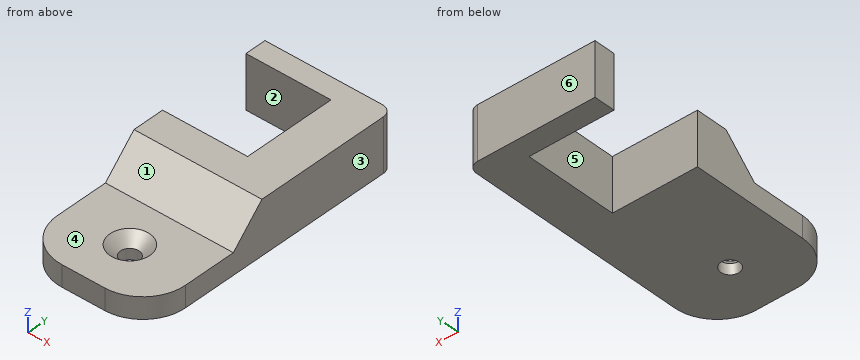
```python
from build123d import *

# Parameters (mm, degrees)
PAD_DEPTH    = 10
SKETCH001_W  = 24.062258
SKETCH001_H  = 24.062258
PAD001_DEPTH = 4
SKETCH002_R  = 1.75
POCKET_DEPTH = 4.001
CHAMFER_SIZE = 2
FILLET_R     = 8
FILLET001_R  = 2
PAD002_DEPTH = 24.062258


with BuildPart() as part:
    # Sketch → Pad (new body)
    with BuildSketch(Plane.XY):
        Polygon((0, 8.75), (0, 12.75), (24.062258, 12.75), (24.062258, -14.75), (0, -14.75), (0, -8.75), (16, -8.75), (16, 8.75), align=None)
    extrude(amount=PAD_DEPTH)

    # Sketch001 (on Face9 of Pad) → Pad001 (join)
    with BuildSketch(Plane(origin=(0, 0, 0), x_dir=(1, 0, 0), z_dir=(0, 0, -1))):
        with Locations((12.031129, 26.781129)):
            Rectangle(SKETCH001_W, SKETCH001_H)
    extrude(amount=-PAD001_DEPTH)

    # Sketch002 (on Face15 of Pad001) → Pocket (cut, through all)
    with BuildSketch(Plane.XY.offset(4)):
        with Locations((12.031129, -29.039748)):
            Circle(SKETCH002_R)
    extrude(amount=-POCKET_DEPTH, mode=Mode.SUBTRACT)

    # Chamfer
    chamfer_edges = [part.edges().sort_by_distance(p)[0] for p in [
        (10.281129, -29.039748, 4),
    ]]
    chamfer(chamfer_edges, length=CHAMFER_SIZE)

    # Fillet
    fillet_edges = [part.edges().sort_by_distance(p)[0] for p in [
        (0, -38.812258, 2),
        (24.062258, -38.812258, 2),
    ]]
    fillet(fillet_edges, radius=FILLET_R)

    # Fillet001
    fillet001_edges = [part.edges().sort_by_distance(p)[0] for p in [
        (24.062258, 12.75, 5),
    ]]
    fillet(fillet001_edges, radius=FILLET001_R)

    # Sketch003 (on Face12 of Fillet001) → Pad002 (join)
    with BuildSketch(Plane.YZ.offset(24.062258)):
        Polygon((-20.75, 4), (-14.75, 10), (-14.75, 4), align=None)
    extrude(amount=-PAD002_DEPTH)


solid = part.part
```
Geometry check sheet. Reference: the model listing, model coordinates, mm. Face numbers are marked on the shaded views. A direction names the side the tool comes from. Give positions to 0.01 mm unless a question says otherwise; leave off trailing zeros. Write each loop counter-clockwise with the first axis right and the second up, starting at its lowest first coordinate (ties: lowest second). Pieces come first, ordered by that corner, then holes. Notation, with made-up numbers: (-1.75, 65) - (50.25, 65) arc R9 ccw to (50.25, 72) - close; hole circle Ø1 at (81.5, 76). An arc over 180 degrees is marked (long way). Use a Markdown table: item, result.
Q1. Set-up check for the marked faces 4, 5 and 6: record each of +Z, -Z, +X, -X, +Y, -Y from which the full face is reachable in a straight line by a thin tool's end or side.
Computed:
| item | result |
|---|---|
| face 4 | +Z, +X, -X, -Y |
| face 5 | +Z, -Z, -X |
| face 6 | +Z, -Z, +X, -X, +Y |
Q2. Section check B-B, the plane x = 3.5. Enter the section's corners in (y, z).
Computed:
| item | result |
|---|---|
| outline | (-37.43, 0) - (-8.75, 0) - (-8.75, 10) - (-14.75, 10) - (-20.75, 4) - (-37.43, 4) - close; (8.75, 0) - (12.75, 0) - (12.75, 10) - (8.75, 10) - close |
Q3. Section check D-D, the plane y = -16. Enter the section's corners in (x, z), then the cut area to 3 significant figures.
Computed:
| item | result |
|---|---|
| outline | (0, 0) - (24.06, 0) - (24.06, 8.75) - (0, 8.75) - close |
| area | 211 mm² |
Q4. Draft check along Y on the marked faces 1, 2 and 3. Enter one of: pulls with the +Y half, pulls with the -Y half, needs draft (parallel to the pull), parting line crosses it, or undercut.
Computed:
| item | result |
|---|---|
| face 1 | pulls with the -Y half |
| face 2 | undercut |
| face 3 | needs draft |
Q5. Section check C-C, the plane z = 1.5. Enter the section's corners in (x, y), then the cut area to 3 significant figures.
Computed:
| item | result |
|---|---|
| outline | (0, -30.81) arc R8 ccw to (8, -38.81) - (16.06, -38.81) arc R8 ccw to (24.06, -30.81) - (24.06, 10.75) arc R2 ccw to (22.06, 12.75) - (0, 12.75) - (0, 8.75) - (16, 8.75) - (16, -8.75) - (0, -8.75) - close; hole circle Ø3.5 at (12.03, -29.04) |
| area | 923 mm² |
Q6. Section check A-A, the plane z = 8. Enter the section's corners in (x, y), then the cut area to 3 significant figures.
Computed:
| item | result |
|---|---|
| outline | (0, -16.75) - (24.06, -16.75) - (24.06, 10.75) arc R2 ccw to (22.06, 12.75) - (0, 12.75) - (0, 8.75) - (16, 8.75) - (16, -8.75) - (0, -8.75) - close |
| area | 429 mm² |
Q7. Go/stop test with flat-tipped pins: P1, Ø4.5, axis at x = 12.03, y = -29.04, coming from the +Z side; P2, Ø5, axis at x = 12, z = 7, coming from the -Y side; P3, Ø1.5, axis at x = 18, y = -19.5, coming from the +Z side. Record where each tip stops, or that it passes through.
Computed:
| item | result |
|---|---|
| P1 | stops at z = 2.5 |
| P2 | stops at y = -20.25 |
| P3 | stops at z = 6 |
Q8. Thickness scan on L1, parallel to Y at x = 14, z = 3; L2, parallel to X at y = 5.5, z = 1.5; L3, parallel to Z at x = 6.25, y = -22. Record the ranges inside material, lowest first. Write a range as [from, to].
Computed:
| item | result |
|---|---|
| L1 | y = [-38.81, -30.96], [-27.12, -8.75], [8.75, 12.75] |
| L2 | x = [16, 24.06] |
| L3 | z = [0, 4] |
